The figure shows three views and two pictorial views of one solid part (mm, origin at its lowest corner). Answer the questions. Round coordinates to 2 decimals unless told otherwise and drop trailing zeros. Order: outer loops, then holes, each group sorted by start corner. A loop starts at its lowest first (then second) coordinate and runs counter-clockwise, first axis right, second up. Notation, with made-up numbers: (44.5, 54) - (95.5, 54) arc R32 cw to (95.5, 88) - close; hole circle Ø1 at (43.5, -2). An arc over 180 degrees is marked (long way). One line per item, written item: value. Start each with the question number.
1. Section C-C, the plane x = 10.5 is taken. Give the vertices of the cut face in (y, z), then the cut area to 3 significant figures.
2. Flat-ended cylindrical pins translate along their axes: P1, Ø1.5, axis at x = 137, y = 22.5, coming from the -Z side; P2, Ø4, axis at x = 150, y = 72.5, coming from the -Z side. Find the tip coordinate at first contact, or state that the pin passes through.
3. Section A-A, the plane y = 66.35 is taken. Give the vertices of the cut face in (x, z), then the cut area to 4 significant figures.
4. Section B-B, the plane x = 30 is taken. Give the vertices of the cut face in (y, z), then the cut area to 3 significant figures.
5. Straight lines are drawn through the part: line 1 (X direction, y = 72.5, z = 1.55); line 2 (Y direction, x = 150, z = 1.6); line 3 (X direction, y = 18.5, z = 3.05). For each, find the intervals that lie inside material, in ascending order.
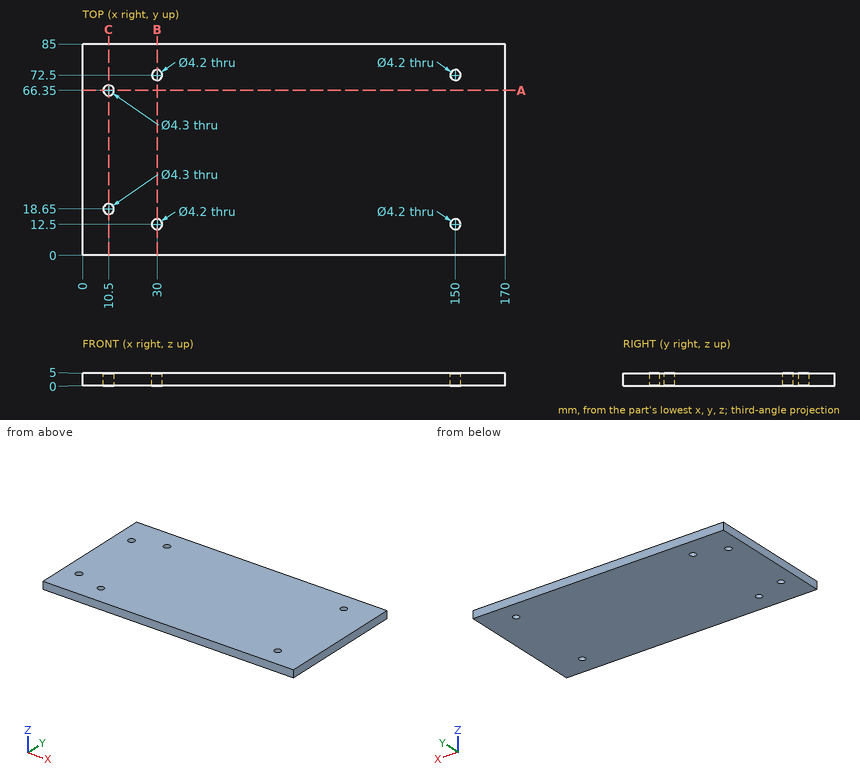
Answer list:
1. outline: (0, 0) - (16.5, 0) - (16.5, 5) - (0, 5) - close; (20.8, 0) - (64.2, 0) - (64.2, 5) - (20.8, 5) - close; (68.5, 0) - (85, 0) - (85, 5) - (68.5, 5) - close
1. area: 382 mm²
2. P1: stops at z = 0
2. P2: passes through
3. outline: (0, 0) - (8.35, 0) - (8.35, 5) - (0, 5) - close; (12.65, 0) - (170, 0) - (170, 5) - (12.65, 5) - close
3. area: 828.5 mm²
4. outline: (0, 0) - (10.4, 0) - (10.4, 5) - (0, 5) - close; (14.6, 0) - (70.4, 0) - (70.4, 5) - (14.6, 5) - close; (74.6, 0) - (85, 0) - (85, 5) - (74.6, 5) - close
4. area: 383 mm²
5. line 1: x = 0 to 27.9, 32.1 to 147.9, 152.1 to 170
5. line 2: y = 0 to 10.4, 14.6 to 70.4, 74.6 to 85
5. line 3: x = 0 to 8.36, 12.64 to 170
